Verification items for this drawing (mm, ordinates from the low corner). Coordinates: 2 decimals unless noted, no trailing zeros. Loops run counter-clockwise (first coordinate to the right, second up) from the corner with the lowest first, then second, coordinate; pieces in that order, holes last. Notation, with made-up numbers: (29, -37) - (52, -37) arc R25 cw to (52, -24) - close; hole circle Ø9 at (-2.5, -9.5). An arc over 180 degrees is marked (long way). Write each question's results on one line, items separated by ' | '. Start each with the question number.
(1) Sectioned sample at B-B (z = 3.25). Enter the section's corners in (x, y), plus the area to 3 significant figures.
(2) Material ranges on probe 1 along X at (y, z) = (54, 10.5); probe 2 along X at (y, z) = (72, 4.5); probe 3 along X at (y, z) = (68, 5.25), recorded low to high.
(3) Go/stop test with flat-tipped pins: pin 1 Ø2 at (x, z) = (67.5, 11) entering from +Y; pin 2 Ø3.5 at (x, z) = (291.5, 5) entering from +Y; pin 3 Ø3.5 at (x, z) = (112.5, 3.5) entering from +Y. Record where each tip stops, or that it passes through.
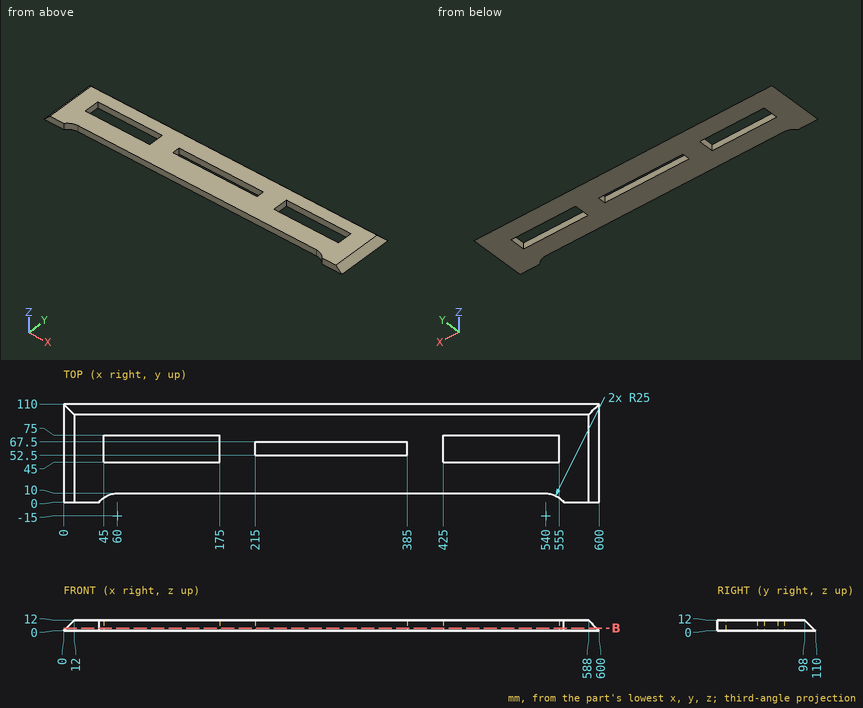
Outcome:
1) outline: (3.25, 0) - (40, 0) arc R25 cw to (60, 10) - (540, 10) arc R25 cw to (560, 0) - (596.75, 0) - (596.75, 106.75) - (3.25, 106.75) - close; hole (45, 45) - (175, 45) - (175, 75) - (45, 75) - close; hole (215, 52.5) - (385, 52.5) - (385, 67.5) - (215, 67.5) - close; hole (425, 45) - (555, 45) - (555, 75) - (425, 75) - close | area: 47,900 mm2
2) probe 1: x = 10.5 to 45, 175 to 215, 385 to 425, 555 to 589.5 | probe 2: x = 4.5 to 45, 175 to 425, 555 to 595.5 | probe 3: x = 5.25 to 45, 175 to 425, 555 to 594.75
3) pin 1: stops at y = 100 | pin 2: stops at y = 106.75 | pin 3: stops at y = 108.25
